Can you work these out from the model? Positions are in its coordinate system, mm. Face numbers are marked on the shaded views. A direction names the side the tool comes from. Coordinates: 2 decimals unless noted, no trailing zeros. Loops run counter-clockwise (first coordinate to the right, second up) from the corner with the lowest first, then second, coordinate; pieces in that order, holes last.
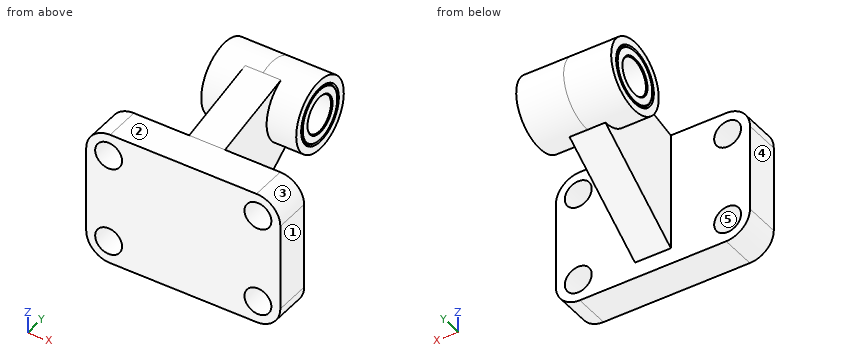
```python
from build123d import *

# Parameters (mm, degrees)
BOSS_EXTRUDE1_DEPTH      = 12
BOSS_EXTRUDE2_DEPTH      = 6
BOSS_EXTRUDE2_DEPTH_BACK = 6
SKETCH3_R                = 12
BOSS_EXTRUDE3_DEPTH      = 15.9
BOSS_EXTRUDE3_DEPTH_BACK = 15.9
SKETCH4_W                = 4.5
SKETCH4_H                = 12
SKETCH5_W                = 4.5
SKETCH5_H                = 12
SKETCH6_W                = 4.5
SKETCH6_H                = 12
SKETCH7_W                = 4.5
SKETCH7_H                = 12


with BuildPart() as part:
    # Sketch1 → Boss-Extrude1 (new body)
    with BuildSketch(Plane(origin=(0, 0, 0), x_dir=(1, 0, 0), z_dir=(0, 1, 0))):
        with BuildLine():
            Line((-24.5, -22.5), (24.5, -22.5))
            ThreePointArc((24.5, -22.5), (30.156854249, -20.156854249), (32.5, -14.5))
            Line((32.5, -14.5), (32.5, 14.5))
            ThreePointArc((32.5, 14.5), (30.156854249, 20.156854249), (24.5, 22.5))
            Line((24.5, 22.5), (-24.5, 22.5))
            ThreePointArc((-24.5, 22.5), (-30.156854249, 20.156854249), (-32.5, 14.5))
            Line((-32.5, 14.5), (-32.5, -14.5))
            ThreePointArc((-32.5, -14.5), (-30.156854249, -20.156854249), (-24.5, -22.5))
        make_face()
    extrude(amount=BOSS_EXTRUDE1_DEPTH)

    # Sketch2 → Boss-Extrude2 (add, two sides)
    with BuildSketch(Plane(origin=(0, 0, 0), x_dir=(0, 0, -1), z_dir=(1, 0, 0))) as boss_extrude2_sk:
        Polygon((-29.505410526, 42.343766684), (-22.5, 12), (17.106848761, 12), (-7.669916362, 47.384887724), align=None)
    extrude(amount=BOSS_EXTRUDE2_DEPTH)
    extrude(boss_extrude2_sk.sketch, amount=-BOSS_EXTRUDE2_DEPTH_BACK)

    # Sketch3 → Boss-Extrude3 (add, two sides)
    with BuildSketch(Plane(origin=(0, 0, 0), x_dir=(0, 0, -1), z_dir=(1, 0, 0))) as boss_extrude3_sk:
        with Locations((-18, 45)):
            Circle(SKETCH3_R)
    extrude(amount=BOSS_EXTRUDE3_DEPTH)
    extrude(boss_extrude3_sk.sketch, amount=-BOSS_EXTRUDE3_DEPTH_BACK)

    # Sketch4 → Cut-Revolve1 (revolve, cut)
    with BuildSketch(Plane.XY.offset(15)):
        with Locations((-27.25, 6)):
            Rectangle(SKETCH4_W, SKETCH4_H)
    revolve(axis=Axis((-25, 12, 15), (0, -1, 0)), mode=Mode.SUBTRACT)

    # Sketch5 → Cut-Revolve2 (revolve, cut)
    with BuildSketch(Plane.XY.offset(15)):
        with Locations((22.75, 6)):
            Rectangle(SKETCH5_W, SKETCH5_H)
    revolve(axis=Axis((25, 12, 15), (0, -1, 0)), mode=Mode.SUBTRACT)

    # Sketch6 → Cut-Revolve3 (revolve, cut)
    with BuildSketch(Plane.XY.offset(-15)):
        with Locations((-27.25, 6)):
            Rectangle(SKETCH6_W, SKETCH6_H)
    revolve(axis=Axis((-25, 12, -15), (0, -1, 0)), mode=Mode.SUBTRACT)

    # Sketch7 → Cut-Revolve4 (revolve, cut)
    with BuildSketch(Plane.XY.offset(-15)):
        with Locations((22.75, 6)):
            Rectangle(SKETCH7_W, SKETCH7_H)
    revolve(axis=Axis((25, 12, -15), (0, -1, 0)), mode=Mode.SUBTRACT)

    # Sketch8 → Cut-Revolve5 (revolve, cut)
    with BuildSketch(Plane.XY.offset(18)):
        Polygon((-15.9, 45), (-15.9, 54.5), (-15.611324865, 54), (15.611324865, 54), (15.9, 54.5), (15.9, 45), align=None)
    revolve(axis=Axis((15.9, 45, 18), (-1, 0, 0)), mode=Mode.SUBTRACT)

    # Sketch9 → Revolve1 (revolve)
    with BuildSketch(Plane.XY.offset(18)):
        Polygon((-15.9, 51.3), (-15.6, 51), (15.6, 51), (15.9, 51.3), (15.9, 53.7), (15.6, 54), (-15.6, 54), (-15.9, 53.7), align=None)
    revolve(axis=Axis((15.9, 45, 18), (-1, 0, 0)))


solid = part.part
```
(1) I want a section at A-A on x = -8. Write out the boundary of the cut face in (y, z), then the cut area to 3 significant figures.
Check values:
outline: (0, -22.5) - (12, -22.5) - (12, 22.5) - (0, 22.5) - close; circle Ø24 at (45, 18); hole circle Ø12 at (45, 18)
area: 879 mm2
(2) I want a section at D-D on z = 17. State how many separate pieces and enclosed holes the cut face has, then the cut area to 3 significant figures.
Check values:
separate pieces: 4
enclosed holes: 0
area: 1,210 mm2
(3) I want a section at B-B on y = 9. Write out the boundary of the cut face in (x, z).
Check values:
outline: (-32.5, -14.5) arc R8 ccw to (-24.5, -22.5) - (24.5, -22.5) arc R8 ccw to (32.5, -14.5) - (32.5, 14.5) arc R8 ccw to (24.5, 22.5) - (-24.5, 22.5) arc R8 ccw to (-32.5, 14.5) - close; hole circle Ø9 at (-25, -15); hole circle Ø9 at (-25, 15); hole circle Ø9 at (25, -15); hole circle Ø9 at (25, 15)
(4) I want a section at C-C on x = -17. Write out the boundary of the cut face in (y, z).
Check values:
outline: (0, -22.5) - (12, -22.5) - (12, 22.5) - (0, 22.5) - close
(5) If I drill on probe 1 along X at (y, z) = (6, 15); probe 2 along Z at (x, y) = (28, 5); probe 3 along X at (y, z) = (2, 13), over which ranges is the centre line in solid material (lowest first)?
Check values:
probe 1: x = -32.48 to -29.5, -20.5 to 20.5, 29.5 to 32.48
probe 2: z = -21.69 to -18.35, -11.65 to 11.65, 18.35 to 21.69
probe 3: x = -32.5 to -29.03, -20.97 to 20.97, 29.03 to 32.5
(6) I'm going to push flat-ended pins straight in: pin 1 (23.5 mm diameter, centred on y = 45, z = 18, fed in from +X); pin 2 (13.5 mm diameter, centred on x = -13, z = -4, fed in from +Y); pin 3 (10 mm diameter, centred on y = 29.5, z = 7, fed in from +X). Where does each tip first touch, or does it pass through?
Check values:
pin 1: stops at x = 15.9
pin 2: stops at y = 12
pin 3: stops at x = 6
(7) If we mould it in two halves opening along X, with no side actions, what happens to the marked faces 3, 4 and 5? For each: released by +X, released by -X, zero draft, split by the parting line, or undercut.
Check values:
face 3: released by +X
face 4: released by -X
face 5: undercut
(8) Which directions (+Z, -Z, +X, -X, +Y, -Y) give clear straight access to the entire face, cutting with the end or side of a thin tool? Please do the marked faces 1 and 2.
Check values:
face 1: +Z, -Z, +X, +Y, -Y
face 2: +Z, +X, -X, -Y
